Autodesk Inventor part; units mm, degrees
ref_plane "YZ Plane" through (0, 0, 0) normal (1, 0, 0) x (0, 1, 0)
ref_plane "XZ Plane" through (0, 0, 0) normal (0, 1, 0) x (-1, 0, 0)
ref_plane "XY Plane" through (0, 0, 0) normal (0, 0, 1) x (1, 0, 0)
sketch "Boceto1" plane through (0, 0, 0) normal (0, 1, 0) x (-1, 0, 0)
  line L0 (0, -5) -> (0, -110)
  line L1 (-5, -115) -> (-107, -115)
  line L2 (-112, -110) -> (-112, -5)
  line L3 (-107, 0) -> (-5, 0)
  arc A0 (-5, -115) -> (0, -110) centre (-5, -110) ccw
  arc A1 (-107, 0) -> (-112, -5) centre (-107, -5) ccw
  arc A2 (-112, -110) -> (-107, -115) centre (-107, -110) ccw
  arc A3 (0, -5) -> (-5, 0) centre (-5, -5) ccw
  circle A4 centre (-10, -105) radius 2
  circle A5 centre (-101, -105) radius 2
  circle A6 centre (-103, -9) radius 2
  circle A7 centre (-11, -9) radius 2
  point P0 (0, 0)
  dimension "d2" = 5
  dimension "d3" = 5
  dimension "d21" = 4
  dimension "d24" = 4
  dimension "d27" = 4
  dimension "d30" = 4
extrude "Extrusión1" add sketch "Boceto1" along normal blind 3
sketch "Boceto2" plane through (0, 3, 0) normal (0, 1, 0) x (1, 0, 0)
  line L0 (5, 0) -> (107, 0)
  line L1 (107, 115) -> (5, 115)
  line L2 (58.3094, 19) -> (60.6188, 15)
  line L3 (60.6188, 15) -> (58.3094, 11)
  line L4 (58.3094, 11) -> (53.6906, 11)
  line L5 (53.6906, 11) -> (51.3812, 15)
  line L6 (51.3812, 15) -> (53.6906, 19)
  line L7 (53.6906, 19) -> (58.3094, 19)
  line L8 (53.6906, 96) -> (51.3812, 100)
  line L9 (51.3812, 100) -> (53.6906, 104)
  line L10 (53.6906, 104) -> (58.3094, 104)
  line L11 (58.3094, 104) -> (60.6188, 100)
  line L12 (60.6188, 100) -> (58.3094, 96)
  line L13 (58.3094, 96) -> (53.6906, 96)
  line L14 (66, 57.5) -> (66, 12.5)
  line L15 (61, 7.5) -> (51, 7.5)
  line L16 (46, 12.5) -> (46, 102.5)
  line L17 (51, 107.5) -> (61, 107.5)
  line L18 (66, 102.5) -> (66, 57.5)
  arc A0 (46, 12.5) -> (51, 7.5) centre (51, 12.5) ccw
  arc A1 (61, 7.5) -> (66, 12.5) centre (61, 12.5) ccw
  arc A2 (66, 102.5) -> (61, 107.5) centre (61, 102.5) ccw
  arc A3 (51, 107.5) -> (46, 102.5) centre (51, 102.5) ccw
  point P0 (0, 0)
  point P1 (56, 15)
  point P2 (56, 100)
  point P3 (66, 107.5)
  dimension "d42" = 5
extrude "Extrusión2" add sketch "Boceto2" along normal blind 3
sketch "Boceto3" plane through (0, 3, 0) normal (0, 1, 0) x (1, 0, 0)
  line L0 (53.6906, 19) -> (58.3094, 19)
  line L1 (58.3094, 104) -> (53.6906, 104)
  circle A0 centre (56, 15) radius 2
  circle A1 centre (56, 100) radius 2
  point P0 (0, 0)
  dimension "d45" = 4
  dimension "d46" = 4
extrude "Extrusión3" cut sketch "Boceto3" against normal blind 3
properties part number "nuc_case_top"
Check sheet for the modelled part. Datum: model origin and axes. Units: mm. A direction names the side the tool comes from. Coordinates: 2 decimals unless noted, no trailing zeros. Write each loop counter-clockwise with the first axis right and the second up, starting at its lowest first coordinate (ties: lowest second). Pieces come first, ordered by that corner, then holes. Notation, with made-up numbers: (-29.5, 43.25) -> (18.5, 43.25) arc R19 ccw to (18.5, 80.25) -> close; hole circle Ø11 at (24.25, -33.5). An arc over 180 degrees is marked (long way). Use a Markdown table: item, result.
1. Sectioned sample at D-D (z = -9). Enter the section's corners in (x, y), plus the area to 3 significant figures.
Reported:
| item | result |
|---|---|
| outline | (0, 0) -> (9, 0) -> (9, 3) -> (0, 3) -> close; (13, 0) -> (101, 0) -> (101, 3) -> (64.57, 3) -> (64.57, 6) -> (47.43, 6) -> (47.43, 3) -> (13, 3) -> close; (105, 0) -> (112, 0) -> (112, 3) -> (105, 3) -> close |
| area | 363 mm2 |
2. Sectioned sample at B-B (y = 4.55). Enter the section's corners in (x, z), plus the area to 3 significant figures.
Reported:
| item | result |
|---|---|
| outline | (46, -102.5) arc R5 ccw to (51, -107.5) -> (61, -107.5) arc R5 ccw to (66, -102.5) -> (66, -12.5) arc R5 ccw to (61, -7.5) -> (51, -7.5) arc R5 ccw to (46, -12.5) -> close; hole (51.38, -100) -> (53.69, -104) -> (58.31, -104) -> (60.62, -100) -> (58.31, -96) -> (53.69, -96) -> close; hole (51.38, -15) -> (53.69, -19) -> (58.31, -19) -> (60.62, -15) -> (58.31, -11) -> (53.69, -11) -> close |
| area | 1,870 mm2 |
3. Sectioned sample at A-A (x = 56). Enter the section's corners in (y, z).
Reported:
| item | result |
|---|---|
| outline | (0, -115) -> (3, -115) -> (3, -107.5) -> (6, -107.5) -> (6, -104) -> (3, -104) -> (3, -102) -> (0, -102) -> close; (0, -98) -> (3, -98) -> (3, -96) -> (6, -96) -> (6, -19) -> (3, -19) -> (3, -17) -> (0, -17) -> close; (0, -13) -> (3, -13) -> (3, -11) -> (6, -11) -> (6, -7.5) -> (3, -7.5) -> (3, 0) -> (0, 0) -> close |
4. Go/stop test with flat-tipped pins: pin 1 Ø3.5 at (x, z) = (11, -9) entering from -Y; pin 2 Ø1.5 at (x, z) = (68, -58) entering from +Y; pin 3 Ø3.5 at (x, y) = (56.5, 5) entering from -Z; pin 4 Ø1.5 at (x, y) = (58.5, 4.5) entering from +Z. Record where each tip stops, or that it passes through.
Reported:
| item | result |
|---|---|
| pin 1 | passes through |
| pin 2 | stops at y = 3 |
| pin 3 | stops at z = -107.5 |
| pin 4 | stops at z = -7.5 |
5. Tool access check on faces 1 (the flat face through (59.448, 4.479, -102.028)), 2 (the flat face through (56, 4, -7.5)), 3 (the flat face through (66, 4, -58)). Record the directions out of +Z, -Z, +X, -X, +Y, -Y that give a thin tool (end or side, any length) a straight path to the whole face; none if there is none.
Reported:
| item | result |
|---|---|
| face 1 | +Y |
| face 2 | +Z, +X, -X, +Y |
| face 3 | +Z, -Z, +X, +Y |
6. Sectioned sample at C-C (z = -89.5). Enter the section's corners in (x, y), plus the area to 3 significant figures.
Reported:
| item | result |
|---|---|
| outline | (0, 0) -> (112, 0) -> (112, 3) -> (66, 3) -> (66, 6) -> (46, 6) -> (46, 3) -> (0, 3) -> close |
| area | 396 mm2 |
7. Scan lines: line 1 along X through (y, z) = (1.55, -15); line 2 along Z through (x, y) = (10, 1.9); line 3 along Y through (x, z) = (14.5, -12.5). Record each from-to range of solid material in increasing order.
Reported:
| item | result |
|---|---|
| line 1 | x = 0 to 54, 58 to 112 |
| line 2 | z = -115 to -107, -103 to -10.73, -7.27 to 0 |
| line 3 | y = 0 to 3 |
8. Release check for a two-part mould opening along Z. For faces 4 (the flat face through (59.48, 4.48, -98.03)), 5 (the cylindrical face through (47.5, 4.48, -8.93)), 6 (the flat face through (56, 6, -58)) record: pulls with the +Z half, pulls with the -Z half, needs draft (parallel to the pull), parting line crosses it, or undercut.
Reported:
| item | result |
|---|---|
| face 4 | undercut |
| face 5 | pulls with the +Z half |
| face 6 | needs draft |
